Can you work these out from the model? Positions are in its coordinate system, mm. Coordinates: 2 decimals unless noted, no trailing zeros. Order: outer loops, then holes, each group sorted by start corner. A loop starts at its lowest first (then second) coordinate and runs counter-clockwise, first axis right, second up. Notation, with made-up numbers: (70.25, 43) -> (109.25, 43) arc R23 cw to (109.25, 66) -> close; hole circle Ø1 at (73.5, 31). An arc over 180 degrees is marked (long way). Answer in a Markdown table with one row per item. Add a question column.
1. Imagine slicing it at D-D on x = -3.25. Write out the boundary of the cut face in (y, z), plus the area to 3 significant figures.
2. Imagine slicing it at B-B on z = 0. Write out the boundary of the cut face in (x, y), plus the area to 3 significant figures.
3. If I drill on line 1 along Z through (x, y) = (3, -1.25); line 2 along X through (y, z) = (-1.5, -0.3); line 3 along Z through (x, y) = (0, -1.05), over which ranges is the centre line in solid material (lowest first)? Write a range as [from, to].
4. Will these pins go through, and if not, where does the flat tip stop? pin 1 (1.3 mm diameter, centred on x = 0, z = 0, fed in from -Y); pin 2 (1 mm diameter, centred on y = -1, z = -0.5, fed in from -X).
5. Imagine slicing it at C-C on x = 3. Write out the boundary of the cut face in (y, z).
6. Imagine slicing it at A-A on y = -0.4. Write out the boundary of the cut face in (x, z).
from build123d import *

# Parameters (mm, degrees)
F0_R     = 0.5
F0_R_2   = 0.8
F1_DEPTH = 2


with BuildPart() as f1:
    # F0 (on Front) → F1 (new body)
    with BuildSketch(Plane.XZ):
        with BuildLine():
            Line((4.683748, 1.75), (-4.683748, 1.75))
            ThreePointArc((-4.683748, 1.75), (-5, 0), (-4.683748, -1.75))
            Line((-4.683748, -1.75), (4.683748, -1.75))
            ThreePointArc((4.683748, -1.75), (5, 0), (4.683748, 1.75))
        make_face()
        with Locations((-3, 0)):
            Circle(F0_R, mode=Mode.SUBTRACT)
        Circle(F0_R_2, mode=Mode.SUBTRACT)
        with Locations((3, 0)):
            Circle(F0_R, mode=Mode.SUBTRACT)
    extrude(amount=F1_DEPTH)


solid = f1.part
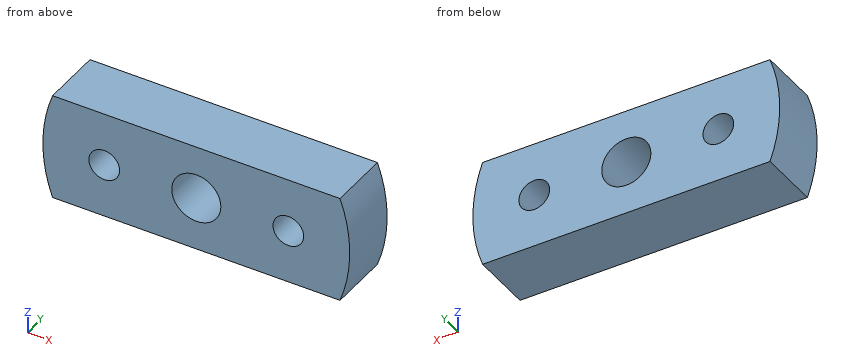
Answers follow:
| question | item | result |
|---|---|---|
| 1 | outline | (-2, -1.75) -> (0, -1.75) -> (0, -0.43) -> (-2, -0.43) -> close; (-2, 0.43) -> (0, 0.43) -> (0, 1.75) -> (-2, 1.75) -> close |
| 1 | area | 5.27 mm² |
| 2 | outline | (-5, -2) -> (-3.5, -2) -> (-3.5, 0) -> (-5, 0) -> close; (-2.5, -2) -> (-0.8, -2) -> (-0.8, 0) -> (-2.5, 0) -> close; (0.8, -2) -> (2.5, -2) -> (2.5, 0) -> (0.8, 0) -> close; (3.5, -2) -> (5, -2) -> (5, 0) -> (3.5, 0) -> close |
| 2 | area | 12.8 mm² |
| 3 | line 1 | z = [-1.75, -0.5], [0.5, 1.75] |
| 3 | line 2 | x = [-4.99, -3.4], [-2.6, -0.74], [0.74, 2.6], [3.4, 4.99] |
| 3 | line 3 | z = [-1.75, -0.8], [0.8, 1.75] |
| 4 | pin 1 | passes through |
| 4 | pin 2 | stops at x = -5 |
| 5 | outline | (-2, -1.75) -> (0, -1.75) -> (0, -0.5) -> (-2, -0.5) -> close; (-2, 0.5) -> (0, 0.5) -> (0, 1.75) -> (-2, 1.75) -> close |
| 6 | outline | (-4.68, -1.75) -> (4.68, -1.75) arc R5 ccw to (4.68, 1.75) -> (-4.68, 1.75) arc R5 ccw to start; hole circle Ø1 at (-3, 0); hole circle Ø1.6 at (0, 0); hole circle Ø1 at (3, 0) |
